The model under review builds one solid part; all positions refer to its coordinate system, in mm. A direction names the side the tool comes from. Coordinates: 2 decimals unless noted, no trailing zeros. Write each loop counter-clockwise with the first axis right and the second up, starting at its lowest first coordinate (ties: lowest second). Pieces come first, ordered by that corner, then holes. Notation, with made-up numbers: (-8, 58.25) - (5, 58.25) arc R20 cw to (5, 71.25) - close; hole circle Ø2 at (-13.75, 64). An arc over 180 degrees is marked (long way). Return JSON: item names as keys, results as strings. Group by question number.
(1) Draft analysis for pull direction X (two halves, no side actions). For faces 1 (the face through (-105.406, -1, 32)), 2 (the face through (-21, 1, 0)), 3 (the face through (15.62, -2.89, 25.86)), state which applies: released by +X, released by -X, zero draft, split by the parting line, or undercut.
(2) For pin 1 Ø19.5 at (y, z) = (19, 37) entering from -X; pin 2 Ø6 at (x, z) = (-83, 36) entering from -Y; pin 3 Ø0.6 at (y, z) = (60, 0.5) entering from +X, all flat-tipped, find the tip position at first contact; note any pin that passes through.
(3) Tool access review of faces 4 (the face through (7.076, -18.913, 25.857)), 5 (the face through (3, 13, 51)): name each direction out of +Z, -Z, +X, -X, +Y, -Y from which nothing blocks a thin tool from reaching the whole face with its end or side.
(4) We need section A-A on y = 20.5. State the section outline as (x, z) points, then the cut area to 3 significant figures.
(5) We need section C-C on z = 9.5. Give the number of separate pieces and of enclosed holes in the cut face, then the cut area to 3 significant figures.
(6) We need section B-B on x = 68. State the section outline as (y, z) points, then the cut area to 3 significant figures.
(7) To check wall thickness, follow L1, parallel to X at y = -42.5, z = 28.5; L2, parallel to Y at x = -114, z = 48.5; L3, parallel to Y at x = -77, z = 32. State the ranges of each line that lie inside material, in increasing order. Write a range as from..to.
```python
from build123d import *

# Parameters (mm, degrees)
ESBO_O1_W                = 210
ESBO_O1_H                = 113
RESSALTO_EXTRUS_O1_DEPTH = 51
ESBO_O2_R                = 2.5
CORTE_EXTRUS_O1_DEPTH    = 51
CORTE_EXTRUS_O2_DEPTH    = 51
ESBO_O4_W                = 18.837176744
ESBO_O4_H                = 106
CORTE_EXTRUS_O3_DEPTH    = 39
ESBO_O5_W                = 6
ESBO_O5_H                = 6
RESSALTO_EXTRUS_O2_DEPTH = 2
ESBO_O6_R                = 1.5
CORTE_EXTRUS_O4_DEPTH    = 148.457044521
ESBO_O7_R                = 1.5
CORTE_EXTRUS_O5_DEPTH    = 148.457044521
ESBO_O8_W                = 6
ESBO_O8_H                = 6
RESSALTO_EXTRUS_O3_DEPTH = 2
ESBO_O9_R                = 1.5
CORTE_EXTRUS_O6_DEPTH    = 148.457044521


with BuildPart() as part:
    # Esboço1 → Ressalto-extrusão1 (new body)
    with BuildSketch(Plane.XY):
        with Locations((-19.243027888, 0)):
            Rectangle(ESBO_O1_W, ESBO_O1_H)
    extrude(amount=RESSALTO_EXTRUS_O1_DEPTH)

    # Esboço2 → Corte-extrusão1 (cut)
    with BuildSketch(Plane.XY.offset(51)):
        with Locations((30.12791278, -9.396028657)):
            Circle(ESBO_O2_R)
        with Locations((22.62791278, -9.396028657)):
            Circle(ESBO_O2_R)
        with Locations((22.62791278, -16.896028657)):
            Circle(ESBO_O2_R)
        with Locations((30.12791278, -16.896028657)):
            Circle(ESBO_O2_R)
        with BuildLine():
            ThreePointArc((33.822919513, -0.400204154), (30.015030071, 1.145986464), (25.930424698, 1.600658183))
            ThreePointArc((25.930424698, 1.600658183), (23.350568744, 4.046940897), (25.796851458, 6.626796851))
            ThreePointArc((25.796851458, 6.626796851), (31.250592932, 6.019721801), (36.334864895, 3.955257029))
            ThreePointArc((36.334864895, 3.955257029), (37.256622795, 0.521553746), (33.822919513, -0.400204154))
        make_face()
        with BuildLine():
            ThreePointArc((35.239711452, 8.890426616), (30.759735868, 10.193403901), (26.112312888, 10.604974905))
            ThreePointArc((26.112312888, 10.604974905), (23.589851495, 13.082309867), (26.067186457, 15.604771261))
            ThreePointArc((26.067186457, 15.604771261), (31.682822558, 15.107456298), (37.096126389, 13.533025412))
            ThreePointArc((37.096126389, 13.533025412), (38.489218319, 10.283518546), (35.239711452, 8.890426616))
        make_face()
        with BuildLine():
            ThreePointArc((41.328918156, -13.387120046), (40.76401379, -9.316295745), (39.115468362, -5.551587868))
            ThreePointArc((39.115468362, -5.551587868), (39.944083361, -2.094225717), (43.401445512, -2.922840715))
            ThreePointArc((43.401445512, -2.922840715), (45.602573834, -7.949456902), (46.356830877, -13.384797967))
            ThreePointArc((46.356830877, -13.384797967), (43.844035556, -15.899915367), (41.328918156, -13.387120046))
        make_face()
        with BuildLine():
            ThreePointArc((33.834918399, -26.380963497), (37.077903475, -23.856329815), (39.513963421, -20.546293656))
            ThreePointArc((39.513963421, -20.546293656), (42.922434373, -19.53521422), (43.933513809, -22.943685172))
            ThreePointArc((43.933513809, -22.943685172), (40.680900657, -27.363226309), (36.350885738, -30.734102602))
            ThreePointArc((36.350885738, -30.734102602), (32.916332516, -29.815516719), (33.834918399, -26.380963497))
        make_face()
        with BuildLine():
            ThreePointArc((18.834919999, -26.387891057), (22.642809441, -27.934081676), (26.727414815, -28.388753395))
            ThreePointArc((26.727414815, -28.388753395), (29.307270768, -30.835036109), (26.860988054, -33.414892062))
            ThreePointArc((26.860988054, -33.414892062), (21.40724658, -32.807817013), (16.322974617, -30.743352241))
            ThreePointArc((16.322974617, -30.743352241), (15.401216717, -27.309648958), (18.834919999, -26.387891057))
        make_face()
        with BuildLine():
            ThreePointArc((11.328921356, -13.400975166), (11.893825722, -17.471799467), (13.54237115, -21.236507344))
            ThreePointArc((13.54237115, -21.236507344), (12.713756151, -24.693869495), (9.256394, -23.865254496))
            ThreePointArc((9.256394, -23.865254496), (7.055265679, -18.838638309), (6.301008635, -13.403297244))
            ThreePointArc((6.301008635, -13.403297244), (8.813803956, -10.888179845), (11.328921356, -13.400975166))
        make_face()
        with BuildLine():
            ThreePointArc((18.822921113, -0.407131715), (15.579936037, -2.931765397), (13.143876092, -6.241801556))
            ThreePointArc((13.143876092, -6.241801556), (9.735405139, -7.252880992), (8.724325703, -3.84441004))
            ThreePointArc((8.724325703, -3.84441004), (11.976938855, 0.575131097), (16.306953774, 3.94600739))
            ThreePointArc((16.306953774, 3.94600739), (19.741506996, 3.027421507), (18.822921113, -0.407131715))
        make_face()
        with BuildLine():
            ThreePointArc((50.08323639, -9.968782472), (48.971660027, -5.437521165), (47.004379482, -1.2069493))
            ThreePointArc((47.004379482, -1.2069493), (47.888583797, 2.216233828), (51.311766925, 1.332029513))
            ThreePointArc((51.311766925, 1.332029513), (53.688897584, -3.77991149), (55.032052356, -9.255185569))
            ThreePointArc((55.032052356, -9.255185569), (52.914442825, -12.086392003), (50.08323639, -9.968782472))
        make_face()
        with BuildLine():
            ThreePointArc((41.172444694, -32.253256694), (44.540843916, -29.024972672), (47.22098635, -25.205971811))
            ThreePointArc((47.22098635, -25.205971811), (50.627652058, -24.260123646), (51.573500224, -27.666789354))
            ThreePointArc((51.573500224, -27.666789354), (48.334994782, -32.281415394), (44.264845723, -36.182258587))
            ThreePointArc((44.264845723, -36.182258587), (40.754144262, -35.763958155), (41.172444694, -32.253256694))
        make_face()
        with BuildLine():
            ThreePointArc((17.41812806, -35.678521828), (21.898103644, -36.981499113), (26.545526624, -37.393070117))
            ThreePointArc((26.545526624, -37.393070117), (29.067988018, -39.870405079), (26.590653055, -42.392866473))
            ThreePointArc((26.590653055, -42.392866473), (20.975016954, -41.89555151), (15.561713123, -40.321120624))
            ThreePointArc((15.561713123, -40.321120624), (14.168621193, -37.071613758), (17.41812806, -35.678521828))
        make_face()
        with BuildLine():
            ThreePointArc((2.574603122, -16.81931274), (3.686179485, -21.350574047), (5.65346003, -25.581145911))
            ThreePointArc((5.65346003, -25.581145911), (4.769255715, -29.00432904), (1.346072587, -28.120124725))
            ThreePointArc((1.346072587, -28.120124725), (-1.031058072, -23.008183722), (-2.374212844, -17.532909643))
            ThreePointArc((-2.374212844, -17.532909643), (-0.256603312, -14.701703209), (2.574603122, -16.81931274))
        make_face()
        with BuildLine():
            ThreePointArc((11.485394818, 5.465161482), (8.116995597, 2.23687746), (5.436853162, -1.582123401))
            ThreePointArc((5.436853162, -1.582123401), (2.030187454, -2.527971566), (1.084339288, 0.878694142))
            ThreePointArc((1.084339288, 0.878694142), (4.32284473, 5.493320182), (8.392993789, 9.394163375))
            ThreePointArc((8.392993789, 9.394163375), (11.90369525, 8.975862943), (11.485394818, 5.465161482))
        make_face()
    extrude(amount=-CORTE_EXTRUS_O1_DEPTH, mode=Mode.SUBTRACT)

    # Esboço3 → Corte-extrusão2 (cut)
    with BuildSketch(Plane.XY.offset(51)):
        with BuildLine():
            Line((-94.441061263, 29.935231702), (-94.441061263, -50.032631861))
            ThreePointArc((-94.441061263, -50.032631861), (-96.941061263, -52.532631861), (-99.441061263, -50.032631861))
            Line((-99.441061263, -50.032631861), (-99.441061263, 29.935231702))
            ThreePointArc((-99.441061263, 29.935231702), (-96.941061263, 32.435231702), (-94.441061263, 29.935231702))
        make_face()
        with BuildLine():
            Line((-84.441061263, 29.935231702), (-84.441061263, -50.032631861))
            ThreePointArc((-84.441061263, -50.032631861), (-86.941061263, -52.532631861), (-89.441061263, -50.032631861))
            Line((-89.441061263, -50.032631861), (-89.441061263, 29.935231702))
            ThreePointArc((-89.441061263, 29.935231702), (-86.941061263, 32.435231702), (-84.441061263, 29.935231702))
        make_face()
        with BuildLine():
            Line((-74.441061263, 29.935231702), (-74.441061263, -50.032631861))
            ThreePointArc((-74.441061263, -50.032631861), (-76.941061263, -52.532631861), (-79.441061263, -50.032631861))
            Line((-79.441061263, -50.032631861), (-79.441061263, 29.935231702))
            ThreePointArc((-79.441061263, 29.935231702), (-76.941061263, 32.435231702), (-74.441061263, 29.935231702))
        make_face()
        with BuildLine():
            Line((-64.441061263, 29.935231702), (-64.441061263, -50.032631861))
            ThreePointArc((-64.441061263, -50.032631861), (-66.941061263, -52.532631861), (-69.441061263, -50.032631861))
            Line((-69.441061263, -50.032631861), (-69.441061263, 29.935231702))
            ThreePointArc((-69.441061263, 29.935231702), (-66.941061263, 32.435231702), (-64.441061263, 29.935231702))
        make_face()
        with BuildLine():
            Line((-54.441061263, 29.935231702), (-54.441061263, -50.032631861))
            ThreePointArc((-54.441061263, -50.032631861), (-56.941061263, -52.532631861), (-59.441061263, -50.032631861))
            Line((-59.441061263, -50.032631861), (-59.441061263, 29.935231702))
            ThreePointArc((-59.441061263, 29.935231702), (-56.941061263, 32.435231702), (-54.441061263, 29.935231702))
        make_face()
    extrude(amount=-CORTE_EXTRUS_O2_DEPTH, mode=Mode.SUBTRACT)

    # Esboço4 → Corte-extrusão3 (cut)
    with BuildSketch(Plane.XY.offset(51)):
        with Locations((-114.824439516, 0)):
            Rectangle(ESBO_O4_W, ESBO_O4_H)
    extrude(amount=-CORTE_EXTRUS_O3_DEPTH, mode=Mode.SUBTRACT)

    # Esboço5 → Ressalto-extrusão2 (add)
    with BuildSketch(Plane.XY):
        with Locations((-95.653704498, 59.5)):
            Rectangle(ESBO_O5_W, ESBO_O5_H)
        with Locations((76.020221531, 59.5)):
            Rectangle(ESBO_O5_W, ESBO_O5_H)
    extrude(amount=RESSALTO_EXTRUS_O2_DEPTH)

    # Esboço6 → Corte-extrusão4 (cut, through all)
    with BuildSketch(Plane.XY.offset(2)):
        with Locations((-95.653704498, 59.5)):
            Circle(ESBO_O6_R)
    extrude(amount=-CORTE_EXTRUS_O4_DEPTH, mode=Mode.SUBTRACT)

    # Esboço7 → Corte-extrusão5 (cut, through all)
    with BuildSketch(Plane.XY.offset(2)):
        with Locations((76.020221531, 59.5)):
            Circle(ESBO_O7_R)
    extrude(amount=-CORTE_EXTRUS_O5_DEPTH, mode=Mode.SUBTRACT)

    # Esboço8 → Ressalto-extrusão3 (add)
    with BuildSketch(Plane.XY):
        with Locations((-95.653027888, -59.5)):
            Rectangle(ESBO_O8_W, ESBO_O8_H)
        with Locations((76.016972112, -59.5)):
            Rectangle(ESBO_O8_W, ESBO_O8_H)
    extrude(amount=RESSALTO_EXTRUS_O3_DEPTH)

    # Esboço9 → Corte-extrusão6 (cut, through all)
    with BuildSketch(Plane.XY.offset(2)):
        with Locations((-95.653027888, -59.5)):
            Circle(ESBO_O9_R)
        with Locations((76.016972112, -59.5)):
            Circle(ESBO_O9_R)
    extrude(amount=-CORTE_EXTRUS_O6_DEPTH, mode=Mode.SUBTRACT)


solid = part.part
```
Ans:
{
 "1": {"face 1": "released by -X", "face 2": "zero draft", "face 3": "undercut"},
 "2": {"pin 1": "x = -105.41", "pin 2": "y = -56.5", "pin 3": "x = 79.02"},
 "3": {"face 4": "+Z, -Z", "face 5": "+Z, +X, -X, +Y, -Y"},
 "4": {"outline": "(-124.24, 0) - (-99.44, 0) - (-99.44, 51) - (-105.41, 51) - (-105.41, 12) - (-124.24, 12) - close; (-94.44, 0) - (-89.44, 0) - (-89.44, 51) - (-94.44, 51) - close; (-84.44, 0) - (-79.44, 0) - (-79.44, 51) - (-84.44, 51) - close; (-74.44, 0) - (-69.44, 0) - (-69.44, 51) - (-74.44, 51) - close; (-64.44, 0) - (-59.44, 0) - (-59.44, 51) - (-64.44, 51) - close; (-54.44, 0) - (85.76, 0) - (85.76, 51) - (-54.44, 51) - close", "area": "8,700 mm²"},
 "5": {"separate pieces": "1", "enclosed holes": "21", "area": "20,700 mm²"},
 "6": {"outline": "(-56.5, 0) - (56.5, 0) - (56.5, 51) - (-56.5, 51) - close", "area": "5,760 mm²"},
 "7": {"L1": "-105.41..-99.44, -94.44..-89.44, -84.44..-79.44, -74.44..-69.44, -64.44..-59.44, -54.44..85.76", "L2": "-56.5..-53, 53..56.5", "L3": "-56.5..-52.53, 32.43..56.5"}
}
